Autodesk Inventor part; units mm, degrees
ref_plane "YZ Plane" through (0, 0, 0) normal (1, 0, 0) x (0, 1, 0)
ref_plane "XZ Plane" through (0, 0, 0) normal (0, 1, 0) x (-1, 0, 0)
ref_plane "XY Plane" through (0, 0, 0) normal (0, 0, 1) x (1, 0, 0)
sketch "Sketch1" plane through (0, 0, 0) normal (0, 1, 0) x (-1, 0, 0)
  line L0 (0, 0) -> (-30, 0)
  line L1 (-30, 0) -> (-30, -30)
  line L2 (-30, -30) -> (0, -30)
  line L3 (0, -30) -> (0, 0)
  dimension "d0" = 30
  dimension "d1" = 30
extrude "Extrusion1" add sketch "Sketch1" along normal blind 70
sketch "Sketch2" plane through (0, 70, 0) normal (0, 1, 0) x (1, 0, 0)
  line L0 (0, 30) -> (0, 0) construction
  line L1 (0, 0) -> (30, 0) construction
  line L2 (0, 30) -> (30, 0) construction
  circle A0 centre (15, 15) radius 11.75
  dimension "d4" = 23.5
extrude "Extrusion2" cut sketch "Sketch2" against normal blind 30
sketch "Sketch3" plane through (0, 0, 0) normal (0, -1, 0) x (1, 0, 0)
  line L0 (30, -30) -> (0, -30) construction
  line L1 (30, -30) -> (0, 0) construction
  circle A0 centre (15, -15) radius 11.75
  dimension "d7" = 23.5
extrude "Extrusion3" cut sketch "Sketch3" against normal blind 30
sketch "Sketch4" plane through (0, 0, 0) normal (0, 0, 1) x (1, 0, 0)
  circle A0 centre (15, 60) radius 1.75
  line L0 (0, 70) -> (30, 70)
  circle A1 centre (15, 10) radius 1.75
  line L1 (0, 0) -> (30, 0)
  dimension "d10" = 3.5
  dimension "d11" = 10
  dimension "d12" = 3.5
  dimension "d13" = 10
extrude "Extrusion4" cut sketch "Sketch4" against normal blind 32
sketch "Sketch5" plane through (0, 0, -30) normal (-1, 0, 0) x (0, 0, 1)
  circle A0 centre (15, 60) radius 1.75
  circle A1 centre (15, 10) radius 1.75
  line L0 (0, 70) -> (30, 70)
  line L1 (0, 0) -> (30, 0)
  dimension "d16" = 3.5
  dimension "d17" = 3.5
  dimension "d18" = 10
  dimension "d19" = 10
extrude "Extrusion5" cut sketch "Sketch5" against normal blind 32
fillet "Fillet1" radius 10 4 edges at (30, 35, 0) (30, 35, -30) (0, 35, -30) (0, 35, 0)
properties part number "Rod_Joint_v2"
Part model, mm, in its own coordinate system. A direction names the side the tool comes from. Give positions to 0.01 mm unless a question says otherwise; leave off trailing zeros. Loops run counter-clockwise (first coordinate to the right, second up) from the corner with the lowest first, then second, coordinate; pieces in that order, holes last. Notation, with made-up numbers: (-16.75, 21.5) -> (-12.75, 21.5) arc R29 cw to (-12.75, 55.5) -> close; hole circle Ø2 at (88.25, 18). An arc over 180 degrees is marked (long way). Write each question's results on one line, items separated by ' | '. Start each with the question number.
Q1. Band-saw the part on A-A on x = 15. List the corners of the cut face in (y, z).
Q2. Band-saw the part on D-D on y = 51.5. List the corners of the cut face in (x, z).
Q3. Pull direction Y, two halves, no side cores. Call faces 1 (the face through (22, 70, -25)), 2 (the face through (3.01, 35.49, -27.15)), 3 (the face through (28.29, 58.45, -14.19)), 4 (the face through (15, 30, -15)): +Y half, -Y half, draft (parallel to the pull), parting line (faces both ways), or undercut.
Q4. Wall check: L1, parallel to Y at x = 15, z = -2.6; L2, parallel to Y at x = 14.5, z = -23.5; L3, parallel to X at y = 13, z = -15.5. Give the ranges that are in metal, low to high.
Q5. Pin check, flat tips, straight feed: P1, Ø2, axis at y = 35.5, z = -7, coming from the +X side; P2, Ø7, axis at x = 20, z = -14, coming from the -Y side; P3, Ø4, axis at x = 11.5, z = -21, coming from the +Y side. Stop position of each tip, or through.
Q6. Which spindle directions (+Z, -Z, +X, -X, +Y, -Y) get a long thin tool onto all of the face, cutting with end or side? Do faces 5 (the face through (26.99, 35.49, -2.85)), 6 (the face through (25.854, 14.79, -19.5)), 7 (the face through (15, 40, -15)). Say none if no direction does.
Q7. Band-saw the part on C-C on z = -15. List the corners of the cut face in (x, y), plus the area to 4 significant figures.
Q8. Band-saw the part on B-B on y = 60. List the corners of the cut face in (x, z), plus the area to 3 significant figures.
Results are:
1) outline: (0, -30) -> (8.25, -30) -> (8.25, -26.75) -> (0, -26.75) -> close; (0, -3.25) -> (8.25, -3.25) -> (8.25, 0) -> (0, 0) -> close; (11.75, -30) -> (58.25, -30) -> (58.25, -26.75) -> (40, -26.75) -> (40, -3.25) -> (58.25, -3.25) -> (58.25, 0) -> (11.75, 0) -> (11.75, -3.25) -> (30, -3.25) -> (30, -26.75) -> (11.75, -26.75) -> close; (61.75, -30) -> (70, -30) -> (70, -26.75) -> (61.75, -26.75) -> close; (61.75, -3.25) -> (70, -3.25) -> (70, 0) -> (61.75, 0) -> close
2) outline: (0, -20) arc R10 ccw to (10, -30) -> (20, -30) arc R10 ccw to (30, -20) -> (30, -10) arc R10 ccw to (20, 0) -> (10, 0) arc R10 ccw to (0, -10) -> close; hole circle Ø23.5 at (15, -15)
3) face 1: +Y half | face 2: draft | face 3: undercut | face 4: -Y half
4) L1: y = 0 to 8.25, 11.75 to 58.25, 61.75 to 70 | L2: y = 30 to 40 | L3: x = 0 to 3.26, 26.74 to 30
5) P1: stops at x = 29.8 | P2: stops at y = 30 | P3: stops at y = 40
6) face 5: +Z, +X, +Y, -Y | face 6: -Y | face 7: +Y
7) outline: (0, 0) -> (3.25, 0) -> (3.25, 8.25) -> (0, 8.25) -> close; (0, 11.75) -> (3.25, 11.75) -> (3.25, 30) -> (26.75, 30) -> (26.75, 11.75) -> (30, 11.75) -> (30, 58.25) -> (26.75, 58.25) -> (26.75, 40) -> (3.25, 40) -> (3.25, 58.25) -> (0, 58.25) -> close; (0, 61.75) -> (3.25, 61.75) -> (3.25, 70) -> (0, 70) -> close; (26.75, 0) -> (30, 0) -> (30, 8.25) -> (26.75, 8.25) -> close; (26.75, 61.75) -> (30, 61.75) -> (30, 70) -> (26.75, 70) -> close | area: 644.5 mm²
8) outline: (0, -20) arc R10 ccw to (10, -30) -> (13.25, -30) -> (13.25, -26.62) arc R11.75 cw to (3.38, -16.75) -> (0, -16.75) -> close; (0, -13.25) -> (3.38, -13.25) arc R11.75 cw to (13.25, -3.38) -> (13.25, 0) -> (10, 0) arc R10 ccw to (0, -10) -> close; (16.75, -30) -> (20, -30) arc R10 ccw to (30, -20) -> (30, -16.75) -> (26.62, -16.75) arc R11.75 cw to (16.75, -26.62) -> close; (16.75, -3.38) arc R11.75 cw to (26.62, -13.25) -> (30, -13.25) -> (30, -10) arc R10 ccw to (20, 0) -> (16.75, 0) -> close | area: 334 mm²
